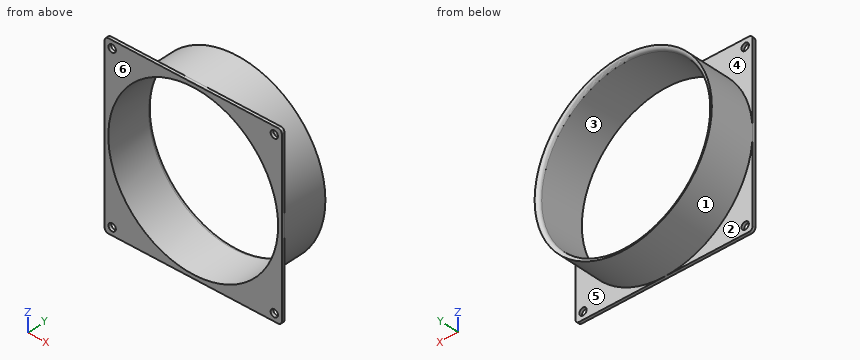
Autodesk Fusion 360 part; units mm, degrees
sketch "Sketch1" plane through (0, 0, 0) normal (0, 1, 0) x (1, 0, 0)
  line L0 (-106.5752, 68.8324) -> (8.4248, 68.8324)
  line L1 (10.9248, 66.3324) -> (10.9248, -48.6676)
  line L2 (8.4248, -51.1676) -> (-106.5752, -51.1676)
  line L3 (-109.0752, -48.6676) -> (-109.0752, 66.3324)
  line L4 (-49.0752, 68.8324) -> (-49.0752, -51.1676)
  line L5 (-109.0752, 8.8324) -> (10.9248, 8.8324)
  circle A0 centre (-49.0752, 8.8324) radius 57.5
  line L6 (-109.0752, 68.8324) -> (-103.9752, 68.8324)
  line L7 (-103.9752, 68.8324) -> (-103.9752, 63.7324)
  circle A1 centre (-103.9752, 63.7324) radius 2.5
  circle A2 centre (5.8248, 63.7324) radius 2.5
  circle A3 centre (-103.9752, -46.0676) radius 2.5
  circle A4 centre (5.8248, -46.0676) radius 2.5
  circle A5 centre (-49.0752, 8.8324) radius 60
  arc A6 (-109.0752, -48.6676) -> (-106.5752, -51.1676) centre (-106.5752, -48.6676) ccw
  arc A7 (8.4248, -51.1676) -> (10.9248, -48.6676) centre (8.4248, -48.6676) ccw
  arc A8 (10.9248, 66.3324) -> (8.4248, 68.8324) centre (8.4248, 66.3324) ccw
  arc A9 (-106.5752, 68.8324) -> (-109.0752, 66.3324) centre (-106.5752, 66.3324) ccw
  point P0 (10.9248, 68.8324)
  point P1 (10.9248, -51.1676)
  dimension "d1" = 120
  dimension "d2" = 120
  dimension "d3" = 115
  dimension "d4" = 5.1
  dimension "d6" = 5.1
  dimension "d7" = 5
  dimension "d8" = 2.5
  dimension "d9" = 2.5
  dimension "d10" = 2.5
  dimension "d11" = 2.5
extrude "Extrude1" add sketch "Sketch1" along normal blind 2 contours L0 L3 L6 A5 A9 | L0 L1 A5 A8 | L2 L3 A5 A6 | L1 L2 A5 A7
extrude "Extrude2" add sketch "Sketch1" along normal blind 24 contours L4 L5 A0 A5 | L4 L5 A0 A5 | L4 L5 A0 A5 | L4 L5 A0 A5
fillet "Fillet1" radius 2 1 edges at (-102.684, 24, -29.6253)
extrude "Extrude3" add sketch "Sketch1" along normal blind 32.3 contours L4 L5 A0 A5 | L4 L5 A0 A5 | L4 L5 A0 A5 | L4 L5 A0 A5
fillet "Fillet2" radius 2.5 1 edges at (-102.684, 32.3, -29.6253)
Geometry: final body of the model. Coordinates: model frame, mm. Face numbers are marked on the shaded views. A direction names the side the tool comes from. Give positions to 0.01 mm unless a question says otherwise; leave off trailing zeros. Loops run counter-clockwise (first coordinate to the right, second up) from the corner with the lowest first, then second, coordinate; pieces in that order, holes last. Notation, with made-up numbers: (81, 63.5) - (119, 63.5) arc R31 ccw to (119, 98.5) - close; hole circle Ø7 at (66, -36). An arc over 180 degrees is marked (long way). One line per question, with ' | ' between items. Start each with the question number.
(1) Section query A-A on y = 7. Return loops of the section in (x, z), then the cut area to 3 significant figures.
(2) Contact query for flat-ended pins moving along their axis: pin 1 (2 mm diameter, centred on y = 20.5, z = 39, fed in from +X); pin 2 (4 mm diameter, centred on x = 5.82, z = -63.73, fed in from +Y); pin 3 (6 mm diameter, centred on x = -65.5, y = 19, fed in from +Z); pin 4 (5 mm diameter, centred on y = 28.5, z = 28.5, fed in from +X). Output: stop coordinate, or through.
(3) Ray query, line 1 (X direction, y = 13.5, z = 12.5); line 2 (Z direction, x = -88, y = 4); line 3 (Z direction, x = -21, y = 26). Return the intervals inside material, ascending. Write a range as from..to.
(4) Reachability of the marked faces 4, 5 and 6 from +Z, -Z, +X, -X, +Y, -Y: full face, straight path, thin tool, end or side. Return the list, or none.
(5) Pull-direction query (X, two-part tool) for the marked faces 1, 2 and 3; classes: released by +X, released by -X, zero draft, split by the parting line, or undercut.
The answers:
1) outline: circle Ø120 at (-49.08, -8.83); hole circle Ø115 at (-49.08, -8.83) | area: 923 mm2
2) pin 1: x = -11.57 | pin 2: through | pin 3: z = 49.65 | pin 4: x = -0.22
3) line 1: -105.15..-102.47, 4.32..7 | line 2: -54.49..-51.15, 33.49..36.83 | line 3: -61.86..-59.01, 41.35..44.19
4) face 4: +Z, -X, +Y | face 5: -Z, +X, +Y | face 6: +Z, -Z, +X, -X, -Y
5) face 1: split by the parting line | face 2: zero draft | face 3: undercut
